from build123d import *

# Parameters (mm, degrees)
SKETCH_1_W           = 140
SKETCH_1_H           = 3
EXTRUDE_1_DEPTH      = 150
CUT_EXTRUDE_1_REACH  = 5
SKETCH_2_W           = 100
SKETCH_2_H           = 100
HOLE_WIZARD_M3_1_D   = 3.4
HOLE_WIZARD_M3_1_2_D = 2


with BuildPart() as part:
    # 草图1 → 拉伸-薄壁1 (new body)
    with BuildSketch(Plane.XY):
        with Locations((82, 225.557982809)):
            Rectangle(SKETCH_1_W, SKETCH_1_H)
    extrude(amount=EXTRUDE_1_DEPTH)

    # 草图2 → 切除-拉伸1 (cut, up to next)
    with BuildSketch(Plane.XZ.offset(-224.057982809), mode=Mode.PRIVATE) as cut_extrude_1_sk1:
        with Locations((82, 75)):
            Rectangle(SKETCH_2_W, SKETCH_2_H)
    cut_extrude_1_tool1 = extrude(cut_extrude_1_sk1.sketch, amount=-CUT_EXTRUDE_1_REACH, mode=Mode.PRIVATE) & part.part
    add(cut_extrude_1_tool1.solids().sort_by_distance((82, 224.057983, 75))[0], mode=Mode.SUBTRACT)

    # Hole Wizard M3 _1 (through all)
    with Locations(Plane(origin=(0, 224.057982809, 0), x_dir=(-1, 0, 0), z_dir=(0, -1, 0))):
        with Locations((-82, -142), (-147, -75), (-82, -8), (-17, -75)):
            Hole(HOLE_WIZARD_M3_1_D / 2)

    # Hole Wizard M3 _1 2 (through all)
    with Locations(Plane(origin=(0, 224.057982809, 0), x_dir=(-1, 0, 0), z_dir=(0, -1, 0))):
        with Locations((-139, -138), (-25, -138), (-82, -130), (-27, -75), (-137, -75), (-82, -20), (-25, -12), (-139, -12)):
            Hole(HOLE_WIZARD_M3_1_2_D / 2)


solid = part.part
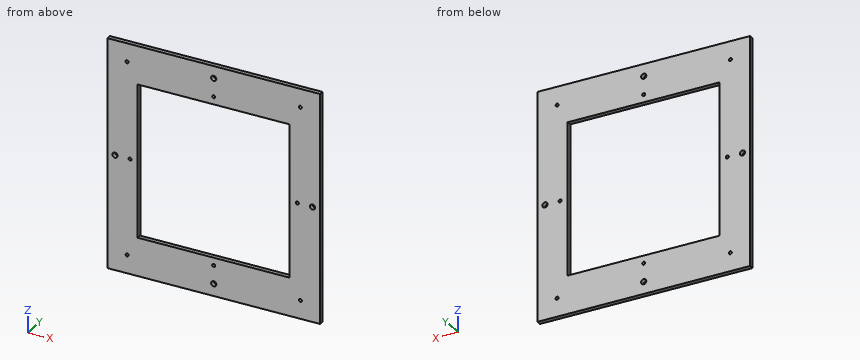
Source: CAD feature listing. Evaluate the final solid. Frame: model axes, mm. Round coordinates to 2 decimals unless told otherwise and drop trailing zeros. Write each loop counter-clockwise with the first axis right and the second up, starting at its lowest first coordinate (ties: lowest second). Pieces come first, ordered by that corner, then holes. Notation, with made-up numbers: (7.25, -36) - (40.25, -36) arc R21 cw to (40.25, -21) - close; hole circle Ø5 at (1, 51.25). An arc over 180 degrees is marked (long way). Use CSV: the item, a comma, the result in double quotes. Start each with the question number.
(1) Cut plane B-B, the plane x = 88. Return loops of the section in (y, z).
(2) Material intervals for probe 1 along X at (y, z) = (224.85, 12); probe 2 along Z at (x, y) = (82, 224.8); probe 3 along Z at (x, y) = (109, 224.4), sorted ascending. Write a range as [from, to].
(3) Cut plane C-C, the plane z = 123. Return loops of the section in (x, y).
(4) First-contact query: pin 1 Ø1.8 at (x, z) = (139, 138) entering from -Y. Flat tip, straight axial feed; report the tip coordinate or a pass-through.
(5) Cut plane A-A, the plane y = 225.1. Give the number of separate pieces and of enclosed holes in the cut face, and give its area (3 significant figures).
Geometry says:
1,outline,"(224.06, 0) - (227.06, 0) - (227.06, 25) - (224.06, 25) - close; (224.06, 125) - (227.06, 125) - (227.06, 150) - (224.06, 150) - close"
2,probe 1,"[12, 24], [26, 138], [140, 152]"
2,probe 2,"[0, 6.3], [9.7, 19], [21, 25], [125, 129], [131, 140.3], [143.7, 150]"
2,probe 3,"[0, 25], [125, 150]"
3,outline,"(12, 224.06) - (32, 224.06) - (32, 227.06) - (12, 227.06) - close; (132, 224.06) - (152, 224.06) - (152, 227.06) - (132, 227.06) - close"
4,pin 1,"through"
5,separate pieces,"1"
5,enclosed holes,"13"
5,area,"10,900 mm²"
